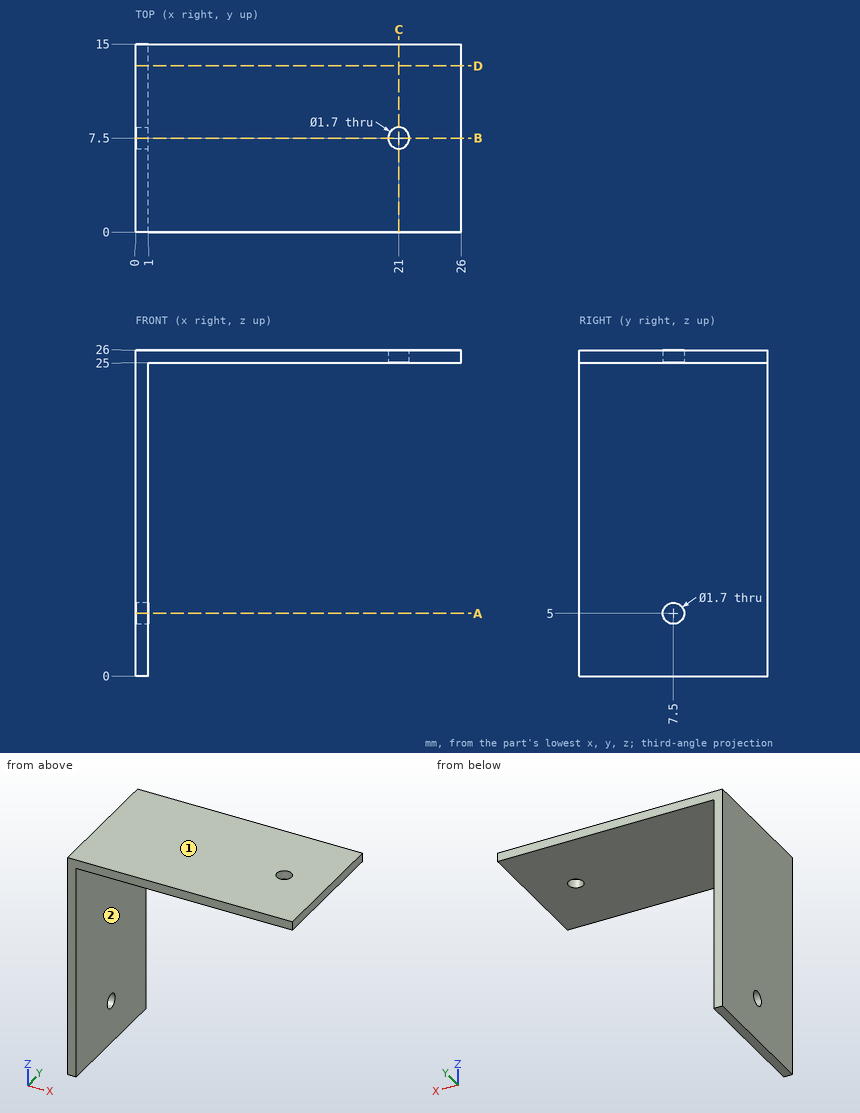
Geometry check sheet. Reference: drawing and pictorial views, mm from the part's lowest x, y, z. A direction names the side the tool comes from. Give positions to 0.01 mm unless a question says otherwise; leave off trailing zeros. Order: outer loops, then holes, each group sorted by start corner. A loop starts at its lowest first (then second) coordinate and runs counter-clockwise, first axis right, second up. Notation, with made-up numbers: M 74,44 L 87,44 A24 cw 87,70 Z; hole C 60,48 d8. An arc over 180 degrees is marked long. Return JSON: item names as keys, results as strings. Group by question number.
1) Scan lines: line 1 (Y direction, x = 0.65, z = 5); line 2 (Z direction, x = 18.25, y = 8.25); line 3 (X direction, y = 10.5, z = 5.5). Record each from-to range of solid material in increasing order.
2) Access from +Z, -Z, +X, -X, +Y, -Y to the whole of each face (thin tool, end or side, straight path). Record for the marked faces 1 and 2.
3) Section check D-D on y = 13.25. Record the cut outline in (x, z), and give its area (3 significant figures).
4) Section check C-C on x = 21. Record the cut outline in (y, z), and give its area (3 significant figures).
5) Section check B-B on y = 7.5. Record the cut outline in (x, z).
6) Go/stop test with flat-tipped pins: pin 1 Ø2 at (y, z) = (7.5, 5) entering from +X; pin 2 Ø5 at (y, z) = (6, 3.5) entering from -X; pin 3 Ø1.5 at (x, y) = (14.5, 7.5) entering from -Z. Record where each tip stops, or that it passes through.
7) Section check A-A on z = 5. Record the cut outline in (x, y), and give its area (3 significant figures).
Answer block:
{
 "1": {"line 1": "y = 0 to 6.65, 8.35 to 15", "line 2": "z = 25 to 26", "line 3": "x = 0 to 1"},
 "2": {"face 1": "+Z, +X, -X, +Y, -Y", "face 2": "-Z, +X, +Y, -Y"},
 "3": {"outline": "M 0,0 L 1,0 L 1,25 L 26,25 L 26,26 L 0,26 Z", "area": "51.0 mm^2"},
 "4": {"outline": "M 0,25 L 6.65,25 L 6.65,26 L 0,26 Z; M 8.35,25 L 15,25 L 15,26 L 8.35,26 Z", "area": "13.3 mm^2"},
 "5": {"outline": "M 0,0 L 1,0 L 1,4.15 L 0,4.15 Z; M 0,5.85 L 1,5.85 L 1,25 L 20.15,25 L 20.15,26 L 0,26 Z; M 21.85,25 L 26,25 L 26,26 L 21.85,26 Z"},
 "6": {"pin 1": "stops at x = 1", "pin 2": "stops at x = 0", "pin 3": "stops at z = 25"},
 "7": {"outline": "M 0,0 L 1,0 L 1,6.65 L 0,6.65 Z; M 0,8.35 L 1,8.35 L 1,15 L 0,15 Z", "area": "13.3 mm^2"}
}
